Part model, mm, in its own coordinate system. Face numbers are marked on the shaded views. A direction names the side the tool comes from. Round coordinates to 2 decimals unless told otherwise and drop trailing zeros. Answer as a JSON object with one key per item and string values. Group by question number.
1. Which spindle directions (+Z, -Z, +X, -X, +Y, -Y) get a long thin tool onto all of the face, cutting with end or side? Do the marked faces 4, 5, 6, 7 and 8. Say none if no direction does.
2. Two-plate mould, pull along X, no slides. Class the marked faces 1, 2 and 3: +X half, -X half, draft (parallel to the pull), parting line (faces both ways), or undercut.
3. Drill centre lines: line 1 (Z direction, x = 0, y = 16.05) (3 decimals); line 2 (Z direction, x = 0, y = -21.55). Where is each one in solid material? Low to high. Write a range as from..to.
4. Drop flat-ended pins along their axis: pin 1 (2 mm diameter, centred on y = -6.5, z = -9, fed in from -X); pin 2 (11.5 mm diameter, centred on x = 0.5, y = 3.5, fed in from +Z); pin 3 (10 mm diameter, centred on y = -0.5, z = -12, fed in from -X) (3 decimals). Give the stop position or say it passes through.
5. Band-saw the part on A-A, the plane x = 0. Count the separate pieces of the cut face and the enclosed holes in it, plus the area to 3 significant figures.
from build123d import *

# Parameters (mm, degrees)
BOSS_EXTRUDE1_DEPTH         = 22.86
BOSS_EXTRUDE1_DEPTH_BACK    = 22.86
SKETCH1_W                   = 45.72
SKETCH1_H                   = 45.72
SKETCH4_R                   = 7.586926628
CUT_EXTRUDE1_DEPTH          = 17.1704
SKETCH5_R                   = 21.442420376
CUT_EXTRUDE2_DEPTH          = 5.715
SKETCH6_R                   = 15.362111806
CUT_EXTRUDE3_DEPTH          = 11.43
CIRPATTERN1_COUNT           = 4
CIRPATTERN2_COUNT           = 2
CIRPATTERN2_ANGLE           = 90
CIRPATTERN2_COPY_1_SKETCH_R = 7.586926628
CIRPATTERN2_COPY_1_DEPTH    = 17.1704
CIRPATTERN2_COPY_2_SKETCH_R = 7.586926628
CIRPATTERN2_COPY_2_DEPTH    = 17.1704
CIRPATTERN2_COPY_3_SKETCH_R = 7.586926628
CIRPATTERN2_COPY_3_DEPTH    = 17.1704
CIRPATTERN2_COPY_4_SKETCH_R = 21.442420376
CIRPATTERN2_COPY_4_DEPTH    = 5.715
CIRPATTERN2_COPY_5_SKETCH_R = 21.442420376
CIRPATTERN2_COPY_5_DEPTH    = 5.715
CIRPATTERN2_COPY_6_SKETCH_R = 21.442420376
CIRPATTERN2_COPY_6_DEPTH    = 5.715
CIRPATTERN2_COPY_7_SKETCH_R = 15.362111806
CIRPATTERN2_COPY_7_DEPTH    = 11.43
CIRPATTERN2_COPY_8_SKETCH_R = 15.362111806
CIRPATTERN2_COPY_8_DEPTH    = 11.43
CIRPATTERN2_COPY_9_SKETCH_R = 15.362111806
CIRPATTERN2_COPY_9_DEPTH    = 11.43


with BuildPart() as part:
    # Sketch1 → Boss-Extrude1 (new, two sides: drawn at the far end of the back side and taken through both)
    with BuildSketch(Plane.XY.offset(-BOSS_EXTRUDE1_DEPTH_BACK)):
        Rectangle(SKETCH1_W, SKETCH1_H)
    extrude(amount=BOSS_EXTRUDE1_DEPTH + BOSS_EXTRUDE1_DEPTH_BACK)

    # Sketch4 → Cut-Extrude1 (cut)
    with BuildSketch(Plane.XY.offset(22.86)):
        Circle(SKETCH4_R)
    cut_extrude1 = extrude(amount=-CUT_EXTRUDE1_DEPTH, mode=Mode.SUBTRACT)

    # Sketch5 → Cut-Extrude2 (cut)
    with BuildSketch(Plane.XY.offset(22.86)):
        Circle(SKETCH5_R)
    cut_extrude2 = extrude(amount=-CUT_EXTRUDE2_DEPTH, mode=Mode.SUBTRACT)

    # Sketch6 → Cut-Extrude3 (cut)
    with BuildSketch(Plane.XY.offset(22.86)):
        Circle(SKETCH6_R)
    cut_extrude3 = extrude(amount=-CUT_EXTRUDE3_DEPTH, mode=Mode.SUBTRACT)

    # CirPattern1: Cut-Extrude1, Cut-Extrude2, Cut-Extrude3 ×4 about axis
    cirpattern1_axis = Axis((0, 0, 0), (0, 1, 0))
    add([cut_extrude1.rotate(cirpattern1_axis, i * 360 / CIRPATTERN1_COUNT) for i in range(1, CIRPATTERN1_COUNT)], mode=Mode.SUBTRACT)
    add([cut_extrude2.rotate(cirpattern1_axis, i * 360 / CIRPATTERN1_COUNT) for i in range(1, CIRPATTERN1_COUNT)], mode=Mode.SUBTRACT)
    add([cut_extrude3.rotate(cirpattern1_axis, i * 360 / CIRPATTERN1_COUNT) for i in range(1, CIRPATTERN1_COUNT)], mode=Mode.SUBTRACT)

    # CirPattern2: Cut-Extrude1, Cut-Extrude2, Cut-Extrude3 ×2 about axis
    cirpattern2_axis = Axis((25.146, 0, 0), (-1, 0, 0))
    add([cut_extrude1.rotate(cirpattern2_axis, i * CIRPATTERN2_ANGLE / (CIRPATTERN2_COUNT - 1)) for i in range(1, CIRPATTERN2_COUNT)], mode=Mode.SUBTRACT)
    add([cut_extrude2.rotate(cirpattern2_axis, i * CIRPATTERN2_ANGLE / (CIRPATTERN2_COUNT - 1)) for i in range(1, CIRPATTERN2_COUNT)], mode=Mode.SUBTRACT)
    add([cut_extrude3.rotate(cirpattern2_axis, i * CIRPATTERN2_ANGLE / (CIRPATTERN2_COUNT - 1)) for i in range(1, CIRPATTERN2_COUNT)], mode=Mode.SUBTRACT)

    # CirPattern2 copy 1 sketch → CirPattern2 copy 1 (cut)
    with BuildSketch(Plane(origin=(22.86, 0, 0), x_dir=(0, -1, 0), z_dir=(1, 0, 0))):
        Circle(CIRPATTERN2_COPY_1_SKETCH_R)
    extrude(amount=-CIRPATTERN2_COPY_1_DEPTH, mode=Mode.SUBTRACT)

    # CirPattern2 copy 2 sketch → CirPattern2 copy 2 (cut)
    with BuildSketch(Plane(origin=(0, -22.86, 0), x_dir=(-1, 0, 0), z_dir=(0, -1, 0))):
        Circle(CIRPATTERN2_COPY_2_SKETCH_R)
    extrude(amount=-CIRPATTERN2_COPY_2_DEPTH, mode=Mode.SUBTRACT)

    # CirPattern2 copy 3 sketch → CirPattern2 copy 3 (cut)
    with BuildSketch(Plane(origin=(-22.86, 0, 0), x_dir=(0, 1, 0), z_dir=(-1, 0, 0))):
        Circle(CIRPATTERN2_COPY_3_SKETCH_R)
    extrude(amount=-CIRPATTERN2_COPY_3_DEPTH, mode=Mode.SUBTRACT)

    # CirPattern2 copy 4 sketch → CirPattern2 copy 4 (cut)
    with BuildSketch(Plane(origin=(22.86, 0, 0), x_dir=(0, -1, 0), z_dir=(1, 0, 0))):
        Circle(CIRPATTERN2_COPY_4_SKETCH_R)
    extrude(amount=-CIRPATTERN2_COPY_4_DEPTH, mode=Mode.SUBTRACT)

    # CirPattern2 copy 5 sketch → CirPattern2 copy 5 (cut)
    with BuildSketch(Plane(origin=(0, -22.86, 0), x_dir=(-1, 0, 0), z_dir=(0, -1, 0))):
        Circle(CIRPATTERN2_COPY_5_SKETCH_R)
    extrude(amount=-CIRPATTERN2_COPY_5_DEPTH, mode=Mode.SUBTRACT)

    # CirPattern2 copy 6 sketch → CirPattern2 copy 6 (cut)
    with BuildSketch(Plane(origin=(-22.86, 0, 0), x_dir=(0, 1, 0), z_dir=(-1, 0, 0))):
        Circle(CIRPATTERN2_COPY_6_SKETCH_R)
    extrude(amount=-CIRPATTERN2_COPY_6_DEPTH, mode=Mode.SUBTRACT)

    # CirPattern2 copy 7 sketch → CirPattern2 copy 7 (cut)
    with BuildSketch(Plane(origin=(22.86, 0, 0), x_dir=(0, -1, 0), z_dir=(1, 0, 0))):
        Circle(CIRPATTERN2_COPY_7_SKETCH_R)
    extrude(amount=-CIRPATTERN2_COPY_7_DEPTH, mode=Mode.SUBTRACT)

    # CirPattern2 copy 8 sketch → CirPattern2 copy 8 (cut)
    with BuildSketch(Plane(origin=(0, -22.86, 0), x_dir=(-1, 0, 0), z_dir=(0, -1, 0))):
        Circle(CIRPATTERN2_COPY_8_SKETCH_R)
    extrude(amount=-CIRPATTERN2_COPY_8_DEPTH, mode=Mode.SUBTRACT)

    # CirPattern2 copy 9 sketch → CirPattern2 copy 9 (cut)
    with BuildSketch(Plane(origin=(-22.86, 0, 0), x_dir=(0, 1, 0), z_dir=(-1, 0, 0))):
        Circle(CIRPATTERN2_COPY_9_SKETCH_R)
    extrude(amount=-CIRPATTERN2_COPY_9_DEPTH, mode=Mode.SUBTRACT)


solid = part.part
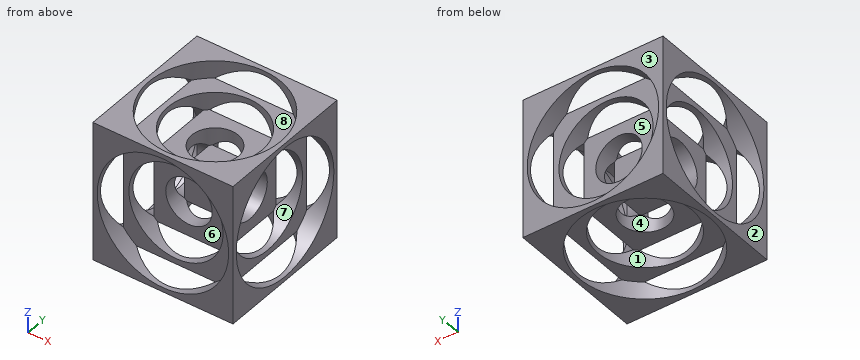
Worked answers:
{
 "1": {"face 4": "-Z", "face 5": "+Y", "face 6": "-Y", "face 7": "+X", "face 8": "+Z"},
 "2": {"face 1": "undercut", "face 2": "-X half", "face 3": "draft"},
 "3": {"line 1": "z = -17.145..-15.362, 15.362..17.145", "line 2": "z = -22.86..-21.44, 21.44..22.86"},
 "4": {"pin 1": "stops at x = -11.43", "pin 2": "stops at z = 11.43", "pin 3": "stops at x = -17.145"},
 "5": {"separate pieces": "13", "enclosed holes": "0", "area": "209 mm^2"}
}
